from build123d import *

# Parameters (mm, degrees)
SKETCH1_W               = 3.2
SKETCH1_H               = 42
EXTRUDE1_DEPTH          = 75
CUT_EXTRUDE1_DEPTH      = 78.900962767
CUT_EXTRUDE1_DEPTH_BACK = 78.900962767
SKETCH2_R               = 1.55
SKETCH2_R_2             = 9.36
SKETCH2_R_3             = 4.6
SKETCH3_R               = 11
CUT_EXTRUDE2_DEPTH      = 2


with BuildPart() as part:
    # Sketch1 → Extrude1 (new body)
    with BuildSketch(Plane.XY):
        Rectangle(SKETCH1_W, SKETCH1_H)
    extrude(amount=EXTRUDE1_DEPTH)

    # Sketch2 → Cut-Extrude1 (cut, two sides: drawn at the far end of the back side and taken through both)
    with BuildSketch(Plane(origin=(0, 0, 0), x_dir=(0, 0, -1), z_dir=(1, 0, 0)).offset(-CUT_EXTRUDE1_DEPTH_BACK)):
        with Locations((-5.5, 15.5)):
            Circle(SKETCH2_R)
        with Locations((-5.5, -15.5)):
            Circle(SKETCH2_R)
        with Locations((-36.5, 15.5)):
            Circle(SKETCH2_R)
        with Locations((-36.5, -15.5)):
            Circle(SKETCH2_R)
        with Locations((-48.36, 0)):
            Circle(SKETCH2_R_2)
        with Locations((-21, 0)):
            Circle(SKETCH2_R_3)
        with BuildLine():
            Line((-36.5, 21), (-58.7375, 6.35))
            ThreePointArc((-58.7375, 6.35), (-60.525927164, 0.072266755), (-58.812204228, -6.226269591))
            Line((-58.812204228, -6.226269591), (-36.5, -21))
            Line((-36.5, -21), (-75, -21))
            Line((-75, -21), (-75, 21))
            Line((-75, 21), (-36.5, 21))
        make_face()
    extrude(amount=CUT_EXTRUDE1_DEPTH + CUT_EXTRUDE1_DEPTH_BACK, mode=Mode.SUBTRACT)

    # Sketch3 → Cut-Extrude2 (cut)
    with BuildSketch(Plane(origin=(1.6, 0, 0), x_dir=(0, 0, -1), z_dir=(1, 0, 0))):
        with Locations((-21, 0)):
            Circle(SKETCH3_R)
    extrude(amount=-CUT_EXTRUDE2_DEPTH, mode=Mode.SUBTRACT)


solid = part.part
For this review, take the finished solid that the model builds, in its own axes (mm). A direction names the side the tool comes from. Give positions to 0.01 mm unless a question says otherwise; leave off trailing zeros. Order: outer loops, then holes, each group sorted by start corner. A loop starts at its lowest first (then second) coordinate and runs counter-clockwise, first axis right, second up. Notation, with made-up numbers: (-19.5, -5.75) - (29.5, -5.75) arc R20 ccw to (29.5, -1.75) - close; hole circle Ø4 at (-3.75, -26). An arc over 180 degrees is marked (long way). Answer as a JSON object with one key per item and string values. Group by question number.
Item 1: Wall thickness on line 1 along Y through (x, z) = (-0.7, 36.5); line 2 along Y through (x, z) = (1.1, 21); line 3 along Z through (x, y) = (0.65, -15.5): over which ranges is each line inside the solid? List them lowest first.
Item 2: Take a section at A-A on z = 21. Give the boundary of the cut face in (x, y).
Item 3: Draft analysis for pull direction Z (two halves, no side actions). For faces 1 (the cylindrical face through (-0.02, 16.81, 35.67)), 2 (the flat face through (-0.02, 13.78, 47.46)), 3 (the flat face through (1.6, 9, 30)), state which applies: pulls with the +Z half, pulls with the -Z half, needs draft (parallel to the pull), parting line crosses it, or undercut.
Item 4: Clearance check with flat-ended pins moving along their axes: pin 1 Ø5 at (y, z) = (-15.5, 5.5) entering from +X; pin 2 Ø1.5 at (x, z) = (0, 49.5) entering from -Y; pin 3 Ø11 at (y, z) = (-5, 19) entering from +X. State where each tip first meets the part, or that it passes through.
Item 5: Take a section at D-D on y = 7.5. Give the boundary of the cut face in (x, z).
Item 6: Take a section at B-B on x = 0.45. Give the boundary of the cut face in (y, z).
Item 7: Machinability: for faces 4 (the flat face through (-0.4, 0, 16)), 5 (the flat face through (-1.6, 4.4, 23.1)), which of the approach directions +Z, -Z, +X, -X, +Y, -Y give a long, thin tool a straight path to every point of the face, cutting with its end or side? Answer none if there is none.
Item 8: Take a section at C-C on y = -4. Give the boundary of the cut face in (x, z), and give its area (3 significant figures).
Reported:
{
 "1": {"line 1": "-21 to -17.05, -13.95 to 13.95, 17.05 to 21", "line 2": "-21 to -11, 11 to 21", "line 3": "0 to 3.95, 7.05 to 34.95, 38.05 to 44.81"},
 "2": {"outline": "(-1.6, -21) - (1.6, -21) - (1.6, -11) - (-0.4, -11) - (-0.4, -4.6) - (-1.6, -4.6) - close; (-1.6, 4.6) - (-0.4, 4.6) - (-0.4, 11) - (1.6, 11) - (1.6, 21) - (-1.6, 21) - close"},
 "3": {"face 1": "undercut", "face 2": "pulls with the +Z half", "face 3": "needs draft"},
 "4": {"pin 1": "x = 1.6", "pin 2": "y = -12.89", "pin 3": "x = -0.4"},
 "5": {"outline": "(-1.6, 0) - (1.6, 0) - (1.6, 12.95) - (-0.4, 12.95) - (-0.4, 29.05) - (1.6, 29.05) - (1.6, 42.76) - (-1.6, 42.76) - close; (-1.6, 53.96) - (1.6, 53.96) - (1.6, 56.99) - (-1.6, 56.99) - close"},
 "6": {"outline": "(-21, 0) - (21, 0) - (21, 36.5) - (6.35, 58.74) arc R12.17 ccw to (-6.23, 58.81) - (-21, 36.5) - close; hole circle Ø3.1 at (-15.5, 5.5); hole circle Ø3.1 at (-15.5, 36.5); hole circle Ø22 at (0, 21); hole circle Ø18.72 at (0, 48.36); hole circle Ø3.1 at (15.5, 5.5); hole circle Ø3.1 at (15.5, 36.5)"},
 "7": {"face 4": "+X", "face 5": "+Z, -Z, -X, +Y, -Y"},
 "8": {"outline": "(-1.6, 0) - (1.6, 0) - (1.6, 10.75) - (-0.4, 10.75) - (-0.4, 18.73) - (-1.6, 18.73) - close; (-1.6, 23.27) - (-0.4, 23.27) - (-0.4, 31.25) - (1.6, 31.25) - (1.6, 39.9) - (-1.6, 39.9) - close; (-1.6, 56.82) - (1.6, 56.82) - (1.6, 59.85) - (-1.6, 59.85) - close", "area": "90.9 mm^2"}
}
